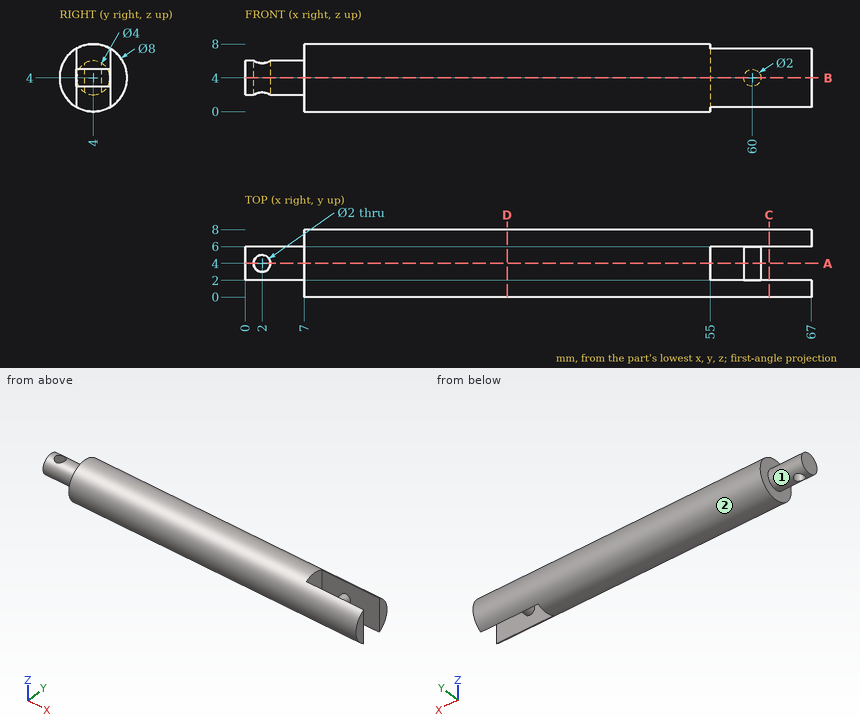
Job drawing, mm, ordinate dimensions from the low corner. One solid piece. A direction names the side the tool comes from. Coordinates: 2 decimals unless noted, no trailing zeros. Write each loop counter-clockwise with the first axis right and the second up, starting at its lowest first coordinate (ties: lowest second). Pieces come first, ordered by that corner, then holes.
Item 1: Slice it at A-A (y = 4). Write the cut outline in (x, z).
Item 2: Which spindle directions (+Z, -Z, +X, -X, +Y, -Y) get a long thin tool onto all of the face, cutting with end or side? Do the marked faces 1 and 2. Say none if no direction does.
Item 3: Slice it at C-C (x = 62). Write the cut outline in (y, z).
Item 4: Pin check, flat tips, straight feed: pin 1 (3 mm diameter, centred on x = 34, z = 6, fed in from +Y); pin 2 (4 mm diameter, centred on x = 7, y = 1.5, fed in from -Z). Stop position of each tip, or through.
Item 5: Slice it at D-D (x = 31). Write the cut outline in (y, z), and give its area (3 significant figures).
Item 6: Probe line 1 (X direction, y = 4, z = 3.85); line 2 (X direction, y = 4, z = 3.6); line 3 (Y direction, x = 2, z = 4.9). List the from-to ranges inside material, lowest first.
Item 7: Slice it at B-B (z = 4). Write the cut outline in (x, y), and give its area (3 significant figures).
Results found:
1. outline: (0, 2) - (1, 2) - (1, 6) - (0, 6) - close; (3, 2) - (7, 2) - (7, 0) - (55, 0) - (55, 8) - (7, 8) - (7, 6) - (3, 6) - close; circle Ø2 at (60, 4)
2. face 1: -X
2. face 2: +X, -X
3. outline: (2, 0.54) - (2, 7.46) arc R4 ccw to start; (6, 0.54) arc R4 ccw to (6, 7.46) - close
4. pin 1: stops at y = 7.97
4. pin 2: stops at z = 0.03
5. outline: circle Ø8 at (4, 4)
5. area: 50.3 mm2
6. line 1: x = 0 to 1, 3 to 55, 59.01 to 60.99
6. line 2: x = 0 to 1, 3 to 55, 59.08 to 60.92
6. line 3: y = 2.21 to 3, 5 to 5.79
7. outline: (0, 2) - (7, 2) - (7, 0) - (67, 0) - (67, 2) - (61, 2) - (61, 6) - (67, 6) - (67, 8) - (7, 8) - (7, 6) - (0, 6) - close; hole circle Ø2 at (2, 4); hole (55, 2) - (59, 2) - (59, 6) - (55, 6) - close
7. area: 465 mm2
